```python
from build123d import *

# Parameters (mm, degrees)
SKICA1_R                 = 1.5
P_IDAT_VYSUNUT_M1_DEPTH  = 3
SKICA3_W                 = 6.5
SKICA3_H                 = 3
P_IDAT_VYSUNUT_M2_DEPTH  = 2
SKICA4_R                 = 1.35
ODEBRAT_VYSUNUT_M1_DEPTH = 3
ZKOSEN_1_SIZE            = 1


with BuildPart() as part:
    # Skica1 → Přidat vysunutím1 (new body)
    with BuildSketch(Plane.XY):
        Polygon((0, 0), (40, 0), (45, 0), (45, 3), (38.5, 3), (16, 48), (0, 48), align=None)
        with Locations((2.5, 22.9)):
            Circle(SKICA1_R, mode=Mode.SUBTRACT)
        with Locations((12.9, 45.1)):
            Circle(SKICA1_R, mode=Mode.SUBTRACT)
        Polygon((3, 3), (35.145898034, 3), (15.37827124, 42.535253588), (3, 18), align=None, mode=Mode.SUBTRACT)
    extrude(amount=P_IDAT_VYSUNUT_M1_DEPTH)

    # Skica3 → Přidat vysunutím2 (add)
    with BuildSketch(Plane(origin=(0, 0, 0), x_dir=(-1, 0, 0), z_dir=(0, 0, -1))):
        with Locations((-41.75, 1.5)):
            Rectangle(SKICA3_W, SKICA3_H)
    extrude(amount=P_IDAT_VYSUNUT_M2_DEPTH)

    # Skica4 → Odebrat vysunutím1 (cut)
    with BuildSketch(Plane(origin=(0, 3, 0), x_dir=(1, 0, 0), z_dir=(0, 1, 0))):
        with Locations((42, -0.5)):
            Circle(SKICA4_R)
    extrude(amount=-ODEBRAT_VYSUNUT_M1_DEPTH, mode=Mode.SUBTRACT)

    # Zkosení1
    zkosen_1_edges = [part.edges().sort_by_distance(p)[0] for p in [
        (40.65, 3, 0.5),
    ]]
    chamfer(zkosen_1_edges, length=ZKOSEN_1_SIZE)


solid = part.part
```
Input: part model. Units: mm. Frame: model coordinates. A direction names the side the tool comes from. Coordinates: 2 decimals unless noted, no trailing zeros. Loops run counter-clockwise (first coordinate to the right, second up) from the corner with the lowest first, then second, coordinate; pieces in that order, holes last. Notation, with made-up numbers: M 80,84 L 107,84 A21 ccw 107,98 Z; hole C -20,84 d8. An arc over 180 degrees is marked long. Use a Markdown table: item, result. Add a question column.
1) Section A-A, the plane x = 42. Return the cut outline in (y, z).
2) Line query: L1, parallel to Z at x = 42, y = 0.7; L2, parallel to Y at x = 2.5, z = 2.25; L3, parallel to X at y = 0.8, z = 0.5. Output: solid intervals per line, ascending. Write a range as from..to.
3) Draft query along X for faces 4 (the flat face through (25.4, 22.49, 1.48)), 5 (the flat face through (0, 24, 1)), 6 (the flat face through (23, 0, 2)). Return one class per face: +X half, -X half, draft (parallel to the pull), parting line (faces both ways), or undercut.
4) Section D-D, the plane z = 1.2. Give the number of separate pieces and of enclosed holes in the cut face, plus the area to 3 significant figures.
5) Section C-C, the plane y = 44.5. Return the cut outline in (x, z), plus the area to 3 significant figures.
6) Section B-B, the plane x = 13. Return the cut outline in (y, z), plus the area to 3 significant figures.
7) Pin query (flat end, axial travel): P1, Ø5, axis at x = 25.5, y = 15.5, coming from the -Z side; P2, Ø2, axis at x = 11.5, y = 38, coming from the -Z side; P3, Ø1.5, axis at x = 21, z = 1.5, coming from the +Y side; P4, Ø2.5, axis at x = 40, z = 0.5, coming from the +Y side. Return the tip coordinate at first contact, or that it passes through.
8) Set-up query: faces 1 (the flat face through (38.5, 1, -1)), 2 (the flat face through (39.6, 3, 1.6)), 3 (the flat face through (19, 3, 1)). Return all of +Z, -Z, +X, -X, +Y, -Y with unobstructed straight access to the full face (end or side cutting, diameter ignored); none if empty.
Answer below:
| question | item | result |
|---|---|---|
| 1 | outline | M 0,-2 L 3,-2 L 3,-1.85 L 2,-0.85 L 0,-0.85 Z; M 0,1.85 L 2,1.85 L 3,2.85 L 3,3 L 0,3 Z |
| 2 | L1 | -2..-0.85, 1.85..3 |
| 2 | L2 | 0..21.4, 24.4..48 |
| 2 | L3 | 0..40.65, 43.35..45 |
| 3 | face 4 | undercut |
| 3 | face 5 | -X half |
| 3 | face 6 | draft |
| 4 | separate pieces | 2 |
| 4 | enclosed holes | 3 |
| 4 | area | 611 mm2 |
| 5 | outline | M 0,0 L 11.53,0 L 11.53,3 L 0,3 Z; M 14.27,0 L 17.75,0 L 17.75,3 L 14.27,3 Z |
| 5 | area | 45.0 mm2 |
| 6 | outline | M 0,0 L 3,0 L 3,3 L 0,3 Z; M 37.82,0 L 43.6,0 L 43.6,3 L 37.82,3 Z; M 46.6,0 L 48,0 L 48,3 L 46.6,3 Z |
| 6 | area | 30.6 mm2 |
| 7 | P1 | through |
| 7 | P2 | z = 0 |
| 7 | P3 | y = 39.5 |
| 7 | P4 | y = 3 |
| 8 | face 1 | -Z, -X, +Y, -Y |
| 8 | face 2 | +Z, -Z, +X, +Y |
| 8 | face 3 | +Z, -Z |
